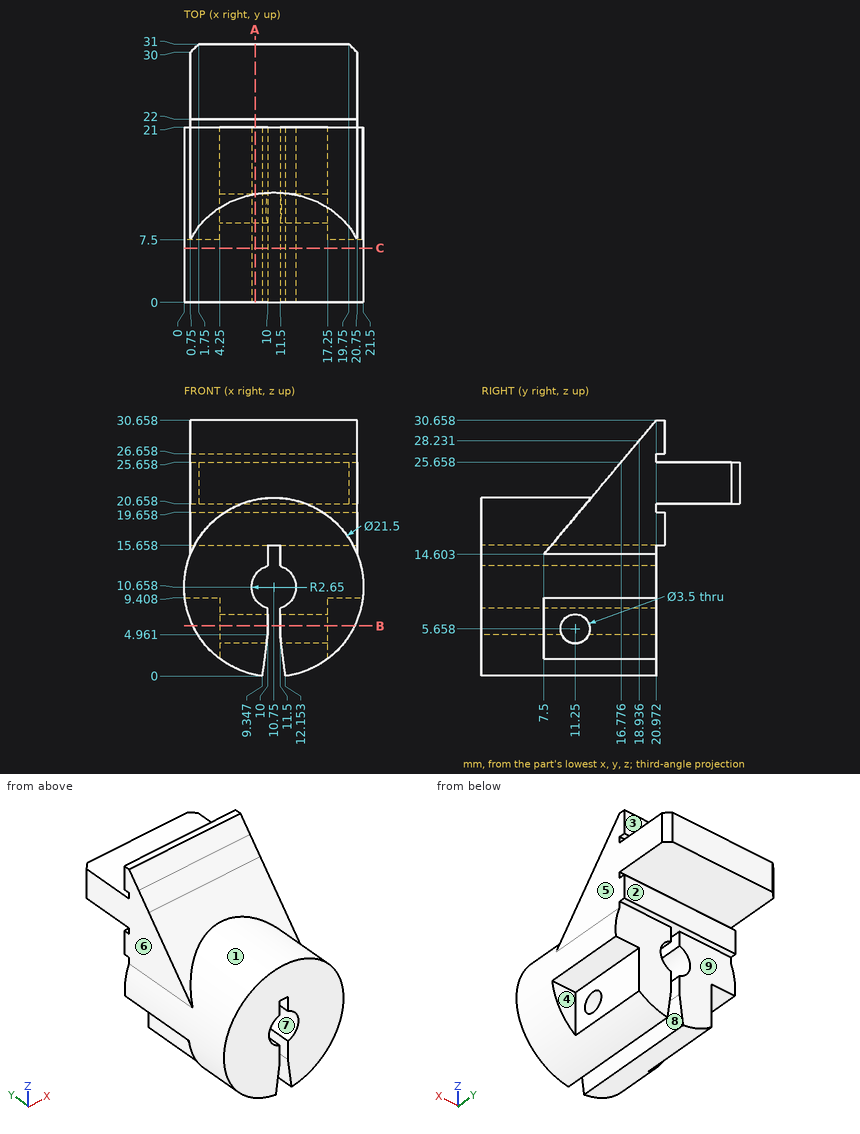
Drawing for the job (mm, zero at the part's lowest x, y, z). A direction names the side the tool comes from. Give positions to 0.01 mm unless a question says otherwise; leave off trailing zeros. Loops run counter-clockwise (first coordinate to the right, second up) from the corner with the lowest first, then second, coordinate; pieces in that order, holes last.
1) Band-saw the part on C-C on y = 6.5. List the corners of the cut face in (x, z).
Values follow:
outline: (9.35, 0) - (10, 4.96) - (10, 8.12) arc R2.65 cw to (10, 13.2) - (10, 15.66) - (11.5, 15.66) - (11.5, 13.2) arc R2.65 cw to (11.5, 8.12) - (11.5, 4.96) - (12.15, 0) arc R10.75 ccw (long way) to start
2) Band-saw the part on A-A on x = 8.5. State how many separate pieces and enclosed holes the cut face has, then the cut area to 3 significant figures.
Values follow:
separate pieces: 2
enclosed holes: 1
area: 469 mm2
3) Probe line 1 along Z through (x, y) = (8.45, 11.25) (1 decimal); line 2 along Z through (x, y) = (5.75, 29); line 3 along Z through (x, y) = (8.7, 11.25) (1 decimal). List the from-to ranges inside material, lowest first.
Values follow:
line 1: z = 0.2 to 3.9, 7.4 to 9.3, 12 to 21.2
line 2: z = 20.66 to 25.66
line 3: z = 0.1 to 3.9, 7.4 to 9, 12.3 to 21.2
4) 3-axis set-ups, long thin cutter, end or side, ignore diameter. For the marked faces 1, 2, 3, 4 and 5: which of +Z, -Z, +X, -X, +Y, -Y reach the whole face in a straight line?
Values follow:
face 1: -Y
face 2: -Z, +X, -X, +Y
face 3: +Z, +X, -X, +Y
face 4: -Z, +X, +Y
face 5: +Z, +X, +Y, -Y
5) Two-plate mould, pull along X, no slides. Class the marked faces 6, 7, 8 and 9: released by +X, released by -X, zero draft, split by the parting line, or undercut.
Values follow:
face 6: released by -X
face 7: undercut
face 8: undercut
face 9: zero draft
6) Band-saw the part on B-B on z = 6. List the corners of the cut face in (x, y).
Values follow:
outline: (1.06, 0) - (10, 0) - (10, 9.53) - (4.25, 9.53) - (4.25, 7.5) - (1.06, 7.5) - close; (4.25, 12.97) - (10, 12.97) - (10, 21) - (4.25, 21) - close; (11.5, 0) - (20.44, 0) - (20.44, 7.5) - (17.25, 7.5) - (17.25, 9.53) - (11.5, 9.53) - close; (11.5, 12.97) - (17.25, 12.97) - (17.25, 21) - (11.5, 21) - close
7) Drop flat-ended pins along their axis: P1, Ø12, axis at y = 17, z = 5, coming from the +X side; P2, Ø3.5, axis at y = 16.5, z = 5, coming from the -X side; P3, Ø10, axis at x = 11, z = 12.5, coming from the +Y side; P4, Ø3, axis at x = 5, y = 17, coming from the -Z side. Give the stop position or say it passes through.
Values follow:
P1: stops at x = 21.5
P2: stops at x = 4.25
P3: stops at y = 22
P4: stops at z = 0.78
